```python
from build123d import *

# Parameters (mm, degrees)
ESBO_O1_R                = 42.5
RESSALTO_EXTRUS_O1_DEPTH = 9
RESSALTO_EXTRUS_O2_START = 2
ESBO_O3_R                = 20.5
ESBO_O3_R_2              = 18.5
RESSALTO_EXTRUS_O2_DEPTH = 2
CORTE_EXTRUS_O1_DEPTH    = 3.2
ESBO_O9_R                = 42.5
ESBO_O9_R_2              = 35.625
RESSALTO_EXTRUS_O4_DEPTH = 0.5
ESBO_O5_R                = 1.5
CORTE_EXTRUS_O2_DEPTH    = 10
PADR_OCIRCULAR1_COUNT    = 6
RESSALTO_EXTRUS_O3_DEPTH = 6
ESBO_O8_R                = 1.5
CORTE_EXTRUS_O3_DEPTH    = 10
PADR_OCIRCULAR2_COUNT    = 4
CHANFRO1_SIZE            = 2


with BuildPart() as part:
    # Esboço1 → Ressalto-extrusão1 (new body)
    with BuildSketch(Plane(origin=(0, 0, 0), x_dir=(1, 0, 0), z_dir=(0, 1, 0))):
        with Locations(Location((0, 0, 0), (0, 0, 270))):
            Circle(ESBO_O1_R)
    extrude(amount=RESSALTO_EXTRUS_O1_DEPTH)

    # Esboço2 → Corte-Revolução1 (revolve, cut)
    with BuildSketch(Plane(origin=(0, 0, 0), x_dir=(0, 0, -1), z_dir=(1, 0, 0))):
        Polygon((0, 0), (-13, 0), (-13, 3.5), (-17, 3.5), (-17, 4), (-18.5, 4), (-18.5, 9), (0, 9), align=None)
    revolve(axis=Axis((0, 9, 0), (0, -1, 0)), mode=Mode.SUBTRACT)

    # Esboço3 → Ressalto-extrusão2 (add)
    with BuildSketch(Plane(origin=(0, 9, 0), x_dir=(1, 0, 0), z_dir=(0, 1, 0)).offset(RESSALTO_EXTRUS_O2_START)):
        with Locations(Location((0, 0, 0), (0, 0, 270))):
            Circle(ESBO_O3_R)
        with Locations(Location((0, 0, 0), (0, 0, 270))):
            Circle(ESBO_O3_R_2, mode=Mode.SUBTRACT)
    extrude(amount=-RESSALTO_EXTRUS_O2_DEPTH)

    # Esboço4 → Corte-extrusão1 (cut)
    with BuildSketch(Plane.XZ):
        with BuildLine():
            Line((-3.75, 39.25), (-3.75, 42.334235555))
            ThreePointArc((-3.75, 42.334235555), (0, 42.5), (3.75, 42.334235555))
            Line((3.75, 42.334235555), (3.75, 39.25))
            ThreePointArc((3.75, 39.25), (0, 35.5), (-3.75, 39.25))
        make_face()
    corte_extrus_o1 = extrude(amount=-CORTE_EXTRUS_O1_DEPTH, mode=Mode.SUBTRACT)

    # Esboço9 → Ressalto-extrusão4 (add)
    with BuildSketch(Plane(origin=(0, 9, 0), x_dir=(1, 0, 0), z_dir=(0, 1, 0))):
        with Locations(Location((0, 0, 0), (0, 0, 275.062092964))):
            Circle(ESBO_O9_R)
        with Locations(Location((0, 0, 0), (0, 0, 270))):
            Circle(ESBO_O9_R_2, mode=Mode.SUBTRACT)
    extrude(amount=RESSALTO_EXTRUS_O4_DEPTH)

    # Esboço5 → Corte-extrusão2 (cut)
    with BuildSketch(Plane.XZ.offset(-3.2)):
        with Locations(Location((0, 39.25, 0), (0, 0, 270))):
            Circle(ESBO_O5_R)
    corte_extrus_o2 = extrude(amount=-CORTE_EXTRUS_O2_DEPTH, mode=Mode.SUBTRACT)

    # PadrãoCircular1: Corte-extrusão1, Corte-extrusão2 ×6 about axis
    padr_ocircular1_axis = Axis((0, 0, 0), (0, 1, 0))
    add([corte_extrus_o1.rotate(padr_ocircular1_axis, i * 360 / PADR_OCIRCULAR1_COUNT) for i in range(1, PADR_OCIRCULAR1_COUNT)], mode=Mode.SUBTRACT)
    add([corte_extrus_o2.rotate(padr_ocircular1_axis, i * 360 / PADR_OCIRCULAR1_COUNT) for i in range(1, PADR_OCIRCULAR1_COUNT)], mode=Mode.SUBTRACT)

    # Esboço6 → Ressalto-extrusão3 (add)
    with BuildSketch(Plane.XZ):
        with BuildLine():
            ThreePointArc((38.890872965, 31.819805153), (38.890872965, 38.890872965), (31.819805153, 38.890872965))
            Line((31.819805153, 38.890872965), (26.30780706, 33.378874872))
            ThreePointArc((26.30780706, 33.378874872), (30.0520382, 30.0520382), (33.378874872, 26.30780706))
            Line((33.378874872, 26.30780706), (38.890872965, 31.819805153))
        make_face()
    ressalto_extrus_o3 = extrude(amount=-RESSALTO_EXTRUS_O3_DEPTH)

    # Esboço8 → Corte-extrusão3 (cut)
    with BuildSketch(Plane.XZ):
        with Locations(Location((35.355339059, 35.355339059, 0), (0, 0, 270))):
            Circle(ESBO_O8_R)
    corte_extrus_o3 = extrude(amount=-CORTE_EXTRUS_O3_DEPTH, mode=Mode.SUBTRACT)

    # PadrãoCircular2: Ressalto-extrusão3, Corte-extrusão3 ×4 about axis
    padr_ocircular2_axis = Axis((0, 0, 0), (0, 1, 0))
    add([ressalto_extrus_o3.rotate(padr_ocircular2_axis, i * 360 / PADR_OCIRCULAR2_COUNT) for i in range(1, PADR_OCIRCULAR2_COUNT)])
    add([corte_extrus_o3.rotate(padr_ocircular2_axis, i * 360 / PADR_OCIRCULAR2_COUNT) for i in range(1, PADR_OCIRCULAR2_COUNT)], mode=Mode.SUBTRACT)

    # Chanfro1
    chanfro1_edges = [part.edges().sort_by_distance(p)[0] for p in [
        (35.355339059, 6, 36.855339059),
        (-36.855339059, 6, 35.355339059),
        (-35.355339059, 6, -36.855339059),
        (36.855339059, 6, -35.355339059),
    ]]
    chamfer(chanfro1_edges, length=CHANFRO1_SIZE)


solid = part.part
```
Here's how the part is built. I have some questions about the finished solid (model axes, mm). A direction names the side the tool comes from. Give positions to 0.01 mm unless a question says otherwise; leave off trailing zeros. Write each loop counter-clockwise with the first axis right and the second up, starting at its lowest first coordinate (ties: lowest second). Pieces come first, ordered by that corner, then holes.
(1) On a 3-axis mill with a long thin cutter (end or side, diameter ignored), from which of +Z, -Z, +X, -X, +Y, -Y can I reach the whole of each face in a straight line? I mean faces 4 (the face through (33.471, 1.578, -23.654)), 5 (the face through (30.786, 1.578, 17.679)), 6 (the face through (-36.17, 2.96, 29.1)). Say none if no direction works.
Output values:
face 4: +X, -Y
face 5: -Y
face 6: -X, +Y, -Y
(2) Imagine slicing it at C-C, the plane z = -10.5. Write out the boundary of the cut face in (x, y).
Output values:
outline: (-41.18, 0) - (-7.66, 0) - (-7.66, 3.5) - (-13.37, 3.5) - (-13.37, 4) - (-15.23, 4) - (-15.23, 11) - (-17.61, 11) - (-17.61, 9) - (-34.04, 9) - (-34.04, 9.5) - (-41.18, 9.5) - close; (7.66, 0) - (41.18, 0) - (41.18, 9.5) - (34.04, 9.5) - (34.04, 9) - (17.61, 9) - (17.61, 11) - (15.23, 11) - (15.23, 4) - (13.37, 4) - (13.37, 3.5) - (7.66, 3.5) - close
(3) If I drill on L1, parallel to X at y = 3.8, z = 0; L2, parallel to Z at x = 34, y = 8.75; L3, parallel to X at y = 8.25, z = 21, over which ranges is the centre line in solid material (lowest first)?
Output values:
L1: x = -42.5 to -17, 17 to 42.5
L2: z = -25.5 to -21.12, -18.13 to 18.13, 21.12 to 25.5
L3: x = -36.95 to -34.59, -33.39 to 33.39, 34.59 to 36.95
(4) Thinking about a two-plate mould opening in Z: for faces 1 (the face through (-35.32, 6.31, -20.32)), 2 (the face through (-0.1, 1.6, -35.5)), 3 (the face through (1, 3.2, -41)), which applies, pulls with the +Z half, pulls with the -Z half, needs draft (parallel to the pull), parting line crosses it, or undercut?
Output values:
face 1: undercut
face 2: pulls with the -Z half
face 3: needs draft
(5) Imagine slicing it at A-A, the plane z = 0. Write out the boundary of the cut face in (x, y) (3 decimals), and give its area (3 significant figures).
Output values:
outline: (-42.5, 0) - (-13, 0) - (-13, 3.5) - (-17, 3.5) - (-17, 4) - (-18.5, 4) - (-18.5, 11) - (-20.5, 11) - (-20.5, 9) - (-35.625, 9) - (-35.625, 9.5) - (-42.5, 9.5) - close; (13, 0) - (42.5, 0) - (42.5, 9.5) - (35.625, 9.5) - (35.625, 9) - (20.5, 9) - (20.5, 11) - (18.5, 11) - (18.5, 4) - (17, 4) - (17, 3.5) - (13, 3.5) - close
area: 487 mm2
(6) Imagine slicing it at D-D, the plane y = 1.75. Count the separate pieces of the cut face and the enclosed holes in it, and give its area (3 significant figures).
Output values:
separate pieces: 1
enclosed holes: 5
area: 5,300 mm2
(7) Imagine slicing it at B-B, the plane z = -30. Write out the boundary of the cut face in (x, y), and give its area (3 significant figures).
Output values:
outline: (-37.07, 0) - (37.07, 0) - (37.07, 6) - (30.1, 6) - (30.1, 9.5) - (19.21, 9.5) - (19.21, 9) - (-19.21, 9) - (-19.21, 9.5) - (-30.1, 9.5) - (-30.1, 6) - (-37.07, 6) - close
area: 636 mm2
(8) Will these pins go through, and if not, where does the flat tip stop? pin 1 (5 mm diameter, centred on y = 9.5, z = 18, fed in from -X); pin 2 (3.5 mm diameter, centred on x = -35.36, z = 35.36, fed in from +Y); pin 3 (4 mm diameter, centred on x = 33.99, z = -19.62, fed in from -Y).
Output values:
pin 1: stops at x = -39.57
pin 2: stops at y = 4.26
pin 3: stops at y = 3.2
